Check sheet for the modelled part. Datum: model origin and axes. Units: mm. Round coordinates to 2 decimals unless told otherwise and drop trailing zeros. Write each loop counter-clockwise with the first axis right and the second up, starting at its lowest first coordinate (ties: lowest second). Pieces come first, ordered by that corner, then holes. Notation, with made-up numbers: M 4.25,31.25 L 23.25,31.25 A22 cw 23.25,41.25 Z; hole C 16,29 d7. An arc over 180 degrees is marked long. Answer in a Markdown table with one row per item.
```python
from build123d import *

# Parameters (mm, degrees)
SKETCH1_W                 = 106.9335
SKETCH1_H                 = 10
BOSS_EXTRUDE1_DEPTH       = 5
FILLET1_RADIUS            = 5
FILLET1_LENGTH            = 5
FILLET2_RADIUS            = 5
FILLET2_LENGTH            = 5
M3X0_5_TAPPED_HOLE1_D     = 2.5
M3X0_5_TAPPED_HOLE1_DEPTH = 29.81
M3X0_5_TAPPED_HOLE1_TIP   = 0.751075774


with BuildPart() as part:
    # Sketch1 → Boss-Extrude1 (new body)
    with BuildSketch(Plane.XY):
        Rectangle(SKETCH1_W, SKETCH1_H)
    extrude(amount=BOSS_EXTRUDE1_DEPTH)

    # Fillet1: full round fillet: the end face becomes a half cylinder, R = half its width
    fillet1_face = Plane((-53.46675, 0, 2.5), x_dir=(0, 0, 1), z_dir=(-1, 0, 0))  # on the end face: x along it, z out of the body
    fillet1_slab = fillet1_face.offset(-FILLET1_RADIUS / 2) * Box(FILLET1_LENGTH, 2 * FILLET1_RADIUS, FILLET1_RADIUS, mode=Mode.PRIVATE)  # the body's end, R deep
    fillet1_round = Plane((-48.46675, 0, 2.5), x_dir=(-1, 0, 0), z_dir=(0, 0, 1)) * Cylinder(FILLET1_RADIUS, FILLET1_LENGTH, mode=Mode.PRIVATE)  # its axis R under the face
    add(fillet1_slab - fillet1_round, mode=Mode.SUBTRACT)

    # Fillet2: full round fillet: the end face becomes a half cylinder, R = half its width
    fillet2_face = Plane((53.46675, 0, 2.5), x_dir=(0, 0, -1), z_dir=(1, 0, 0))  # on the end face: x along it, z out of the body
    fillet2_slab = fillet2_face.offset(-FILLET2_RADIUS / 2) * Box(FILLET2_LENGTH, 2 * FILLET2_RADIUS, FILLET2_RADIUS, mode=Mode.PRIVATE)  # the body's end, R deep
    fillet2_round = Plane((48.46675, 0, 2.5), x_dir=(1, 0, 0), z_dir=(0, 0, -1)) * Cylinder(FILLET2_RADIUS, FILLET2_LENGTH, mode=Mode.PRIVATE)  # its axis R under the face
    add(fillet2_slab - fillet2_round, mode=Mode.SUBTRACT)

    # M3x0.5 Tapped Hole1
    with Locations(Plane.XY.offset(5)):
        with Locations((-48.46675, 0), (48.46675, 0)):
            Hole(M3X0_5_TAPPED_HOLE1_D / 2, depth=M3X0_5_TAPPED_HOLE1_DEPTH)
            with Locations((0, 0, -(M3X0_5_TAPPED_HOLE1_DEPTH + M3X0_5_TAPPED_HOLE1_TIP / 2))):  # 118° drill point
                Cone(0, M3X0_5_TAPPED_HOLE1_D / 2, M3X0_5_TAPPED_HOLE1_TIP, mode=Mode.SUBTRACT)


solid = part.part
```
1. Draft check along X on faces 1 (the face through (-1, 5, 2)), 2 (the face through (-49.659, 0.375, 2.465)), 3 (the face through (53.466, 0.11, 2.465)), 4 (the face through (-53.466, 0.11, 2.535)). Enter one of: +X half, -X half, draft (parallel to the pull), parting line (faces both ways), or undercut.
Found:
| item | result |
|---|---|
| face 1 | draft |
| face 2 | undercut |
| face 3 | +X half |
| face 4 | -X half |
2. Go/stop test with flat-tipped pins: pin 1 (1.5 mm diameter, centred on y = 3.5, z = 3.5, fed in from -X); pin 2 (2 mm diameter, centred on x = 48.47, y = 0, fed in from -Z). Record where each tip stops, or that it passes through.
Found:
| item | result |
|---|---|
| pin 1 | stops at x = -52.64 |
| pin 2 | passes through |
3. Section check B-B, the plane z = 4. Record the cut outline in (x, y), and give its area (3 significant figures).
Found:
| item | result |
|---|---|
| outline | M -48.47,-5 L 48.47,-5 A5 ccw 48.47,5 L -48.47,5 A5 ccw Z; hole C -48.47,0 d2.5; hole C 48.47,0 d2.5 |
| area | 1,040 mm2 |
4. Scan lines: L1, parallel to X at y = -0.5, z = 1.25; L2, parallel to X at y = 0.25, z = 1.6; L3, parallel to X at y = 2.75, z = 3.3. Record each from-to range of solid material in increasing order.
Found:
| item | result |
|---|---|
| L1 | x = -53.44 to -49.61, -47.32 to 47.32, 49.61 to 53.44 |
| L2 | x = -53.46 to -49.69, -47.24 to 47.24, 49.69 to 53.46 |
| L3 | x = -52.64 to 52.64 |
5. Section check A-A, the plane y = 0. Record the cut outline in (x, z).
Found:
| item | result |
|---|---|
| outline | M -53.47,0 L -49.72,0 L -49.72,5 L -53.47,5 Z; M -47.22,0 L 47.22,0 L 47.22,5 L -47.22,5 Z; M 49.72,0 L 53.47,0 L 53.47,5 L 49.72,5 Z |
